Design review of the part built by this model. Coordinates are the model's own, in mm. Give positions to 0.01 mm unless a question says otherwise; leave off trailing zeros. Order: outer loops, then holes, each group sorted by start corner. A loop starts at its lowest first (then second) coordinate and runs counter-clockwise, first axis right, second up. Notation, with made-up numbers: M 8.25,-5 L 58.25,-5 A21 cw 58.25,32 Z; hole C -25.5,22.25 d8. An arc over 180 degrees is marked long. Answer as a JSON object with one key per item and string values.
from build123d import *

# Parameters (mm, degrees)
SKETCH1_W                    = 228.6
SKETCH1_H                    = 50.8
BOSS_EXTRUDE1_DEPTH          = 3.175
F_10_0_1935_DIAMETER_HOLE1_D = 4.9149
F_1_4_20_TAPPED_HOLE1_D      = 5.1054


with BuildPart() as part:
    # Sketch1 → Boss-Extrude1 (new body)
    with BuildSketch(Plane(origin=(0, 0, 0), x_dir=(1, 0, 0), z_dir=(0, 1, 0))):
        Rectangle(SKETCH1_W, SKETCH1_H)
    extrude(amount=BOSS_EXTRUDE1_DEPTH)

    # #10 (0.1935) Diameter Hole1 (through all)
    with Locations(Plane(origin=(0, 3.175, 0), x_dir=(1, 0, 0), z_dir=(0, 1, 0))):
        with Locations((107.95, 12.7), (-101.6, -12.7), (-101.6, 12.7), (107.95, -12.7)):
            Hole(F_10_0_1935_DIAMETER_HOLE1_D / 2)

    # 1/4-20 Tapped Hole1 (through all)
    with Locations(Plane(origin=(0, 3.175, 0), x_dir=(1, 0, 0), z_dir=(0, 1, 0))):
        with Locations((-76.2, -13.97), (-19.05, 13.97)):
            Hole(F_1_4_20_TAPPED_HOLE1_D / 2)


solid = part.part
(1) Draft analysis for pull direction Z (two halves, no side actions). For faces 1 (the cylindrical face through (-99.145, 1.565, -12.808)), 2 (the flat face through (-2, 0, 0)), 3 (the cylindrical face through (-99.65, 1.565, 14.195)), state which applies: +Z half, -Z half, draft (parallel to the pull), parting line (faces both ways), or undercut.
Checked values:
{"face 1": "undercut", "face 2": "draft", "face 3": "undercut"}
(2) To check wall thickness, follow L1, parallel to Z at x = -19.05, y = 0.8; L2, parallel to X at y = 2.1, z = -12.7; L3, parallel to X at y = 0.9, z = 13.97. State the ranges of each line that lie inside material, in increasing order. Write a range as from..to.
Checked values:
{"L1": "z = -25.4..-16.52, -11.42..25.4", "L2": "x = -114.3..-104.06, -99.14..-21.26, -16.84..105.49, 110.41..114.3", "L3": "x = -114.3..-103.7, -99.5..-78.75, -73.65..105.85, 110.05..114.3"}
(3) We need section B-B (x = -101.6). Write out the cut boundary in (y, z) (3 decimals).
Checked values:
{"outline": "M 0,-25.4 L 3.175,-25.4 L 3.175,-15.157 L 0,-15.157 Z; M 0,-10.243 L 3.175,-10.243 L 3.175,10.243 L 0,10.243 Z; M 0,15.157 L 3.175,15.157 L 3.175,25.4 L 0,25.4 Z"}
(4) We need section A-A (x = -19.05). Write out the cut boundary in (y, z) (3 decimals), plus the area to 3 significant figures.
Checked values:
{"outline": "M 0,-25.4 L 3.175,-25.4 L 3.175,-16.523 L 0,-16.523 Z; M 0,-11.417 L 3.175,-11.417 L 3.175,25.4 L 0,25.4 Z", "area": "145 mm^2"}
